Could you check a few things on this drawing? It's one solid part, dimensions in mm from its lowest x, y, z. A direction names the side the tool comes from. Round coordinates to 2 decimals unless told otherwise and drop trailing zeros. Write each loop counter-clockwise with the first axis right and the second up, starting at its lowest first coordinate (ties: lowest second). Pieces come first, ordered by that corner, then holes. Notation, with made-up numbers: (19.5, 64.5) -> (52.5, 64.5) arc R33 cw to (52.5, 92.5) -> close; hole circle Ø8 at (52.5, 16). An arc over 180 degrees is marked (long way). Answer in a Markdown table with one row per item.
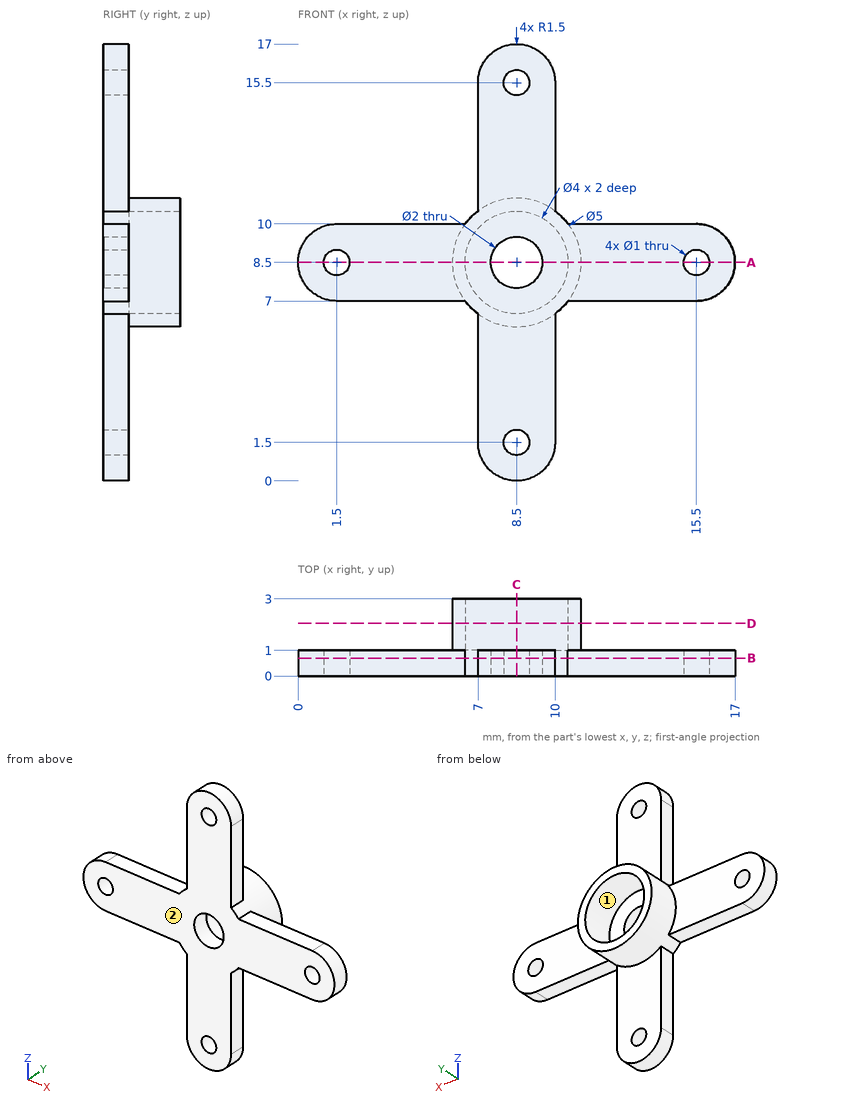
1) Which directions (+Z, -Z, +X, -X, +Y, -Y) give clear straight access to the entire face, cutting with the end or side of a thin tool? Please do the marked faces 1 and 2.
Response:
| item | result |
|---|---|
| face 1 | +Y |
| face 2 | +Z, -Z, +X, -X, -Y |
2) I want a section at C-C, the plane x = 8.5. List the corners of the cut face in (y, z) for me.
Response:
| item | result |
|---|---|
| outline | (0, 0) -> (1, 0) -> (1, 1) -> (0, 1) -> close; (0, 2) -> (1, 2) -> (1, 6) -> (3, 6) -> (3, 6.5) -> (1, 6.5) -> (1, 7.5) -> (0, 7.5) -> close; (0, 9.5) -> (1, 9.5) -> (1, 10.5) -> (3, 10.5) -> (3, 11) -> (1, 11) -> (1, 15) -> (0, 15) -> close; (0, 16) -> (1, 16) -> (1, 17) -> (0, 17) -> close |
3) I want a section at A-A, the plane z = 8.5. List the corners of the cut face in (x, y) for me, and give its area (3 significant figures).
Response:
| item | result |
|---|---|
| outline | (0, 0) -> (1, 0) -> (1, 1) -> (0, 1) -> close; (2, 0) -> (7.5, 0) -> (7.5, 1) -> (6.5, 1) -> (6.5, 3) -> (6, 3) -> (6, 1) -> (2, 1) -> close; (9.5, 0) -> (15, 0) -> (15, 1) -> (11, 1) -> (11, 3) -> (10.5, 3) -> (10.5, 1) -> (9.5, 1) -> close; (16, 0) -> (17, 0) -> (17, 1) -> (16, 1) -> close |
| area | 15.0 mm^2 |
4) For pin 1 (3 mm diameter, centred on x = 8.5, z = 8.5, fed in from +Y); pin 2 (0.5 mm diameter, centred on y = 0.5, z = 12.5, fed in from -X); pin 3 (1 mm diameter, centred on y = 0.5, z = 8, fed in from -X); pin 4 (0.8 mm diameter, centred on x = 5, y = 0.5, fed in from +Z), each with a flat end and sliding along its axis, tell me the tip position at first contact or that it passes through.
Response:
| item | result |
|---|---|
| pin 1 | stops at y = 1 |
| pin 2 | stops at x = 7 |
| pin 3 | stops at x = 0 |
| pin 4 | stops at z = 10 |
5) I want a section at B-B, the plane y = 0.7. List the corners of the cut face in (x, z) for me.
Response:
| item | result |
|---|---|
| outline | (1.5, 7) -> (6.5, 7) arc R2.5 ccw to (7, 6.5) -> (7, 1.5) arc R1.5 ccw to (10, 1.5) -> (10, 6.5) arc R2.5 ccw to (10.5, 7) -> (15.5, 7) arc R1.5 ccw to (15.5, 10) -> (10.5, 10) arc R2.5 ccw to (10, 10.5) -> (10, 15.5) arc R1.5 ccw to (7, 15.5) -> (7, 10.5) arc R2.5 ccw to (6.5, 10) -> (1.5, 10) arc R1.5 ccw to start; hole circle Ø1 at (1.5, 8.5); hole circle Ø2 at (8.5, 8.5); hole circle Ø1 at (8.5, 1.5); hole circle Ø1 at (8.5, 15.5); hole circle Ø1 at (15.5, 8.5) |
6) I want a section at D-D, the plane y = 2.05. List the corners of the cut face in (x, z) for me, and give its area (3 significant figures).
Response:
| item | result |
|---|---|
| outline | circle Ø5 at (8.5, 8.5); hole circle Ø4 at (8.5, 8.5) |
| area | 7.07 mm^2 |
7) I need wall thicknesses on line 1 (X direction, y = 0.75, z = 8.5); line 2 (X direction, y = 0.5, z = 1.5); line 3 (Y direction, x = 2, z = 7.25). Which ranges of each line are inside material? Lowest first, please. Write a range as [from, to].
Response:
| item | result |
|---|---|
| line 1 | x = [0, 1], [2, 7.5], [9.5, 15], [16, 17] |
| line 2 | x = [7, 8], [9, 10] |
| line 3 | y = [0, 1] |
